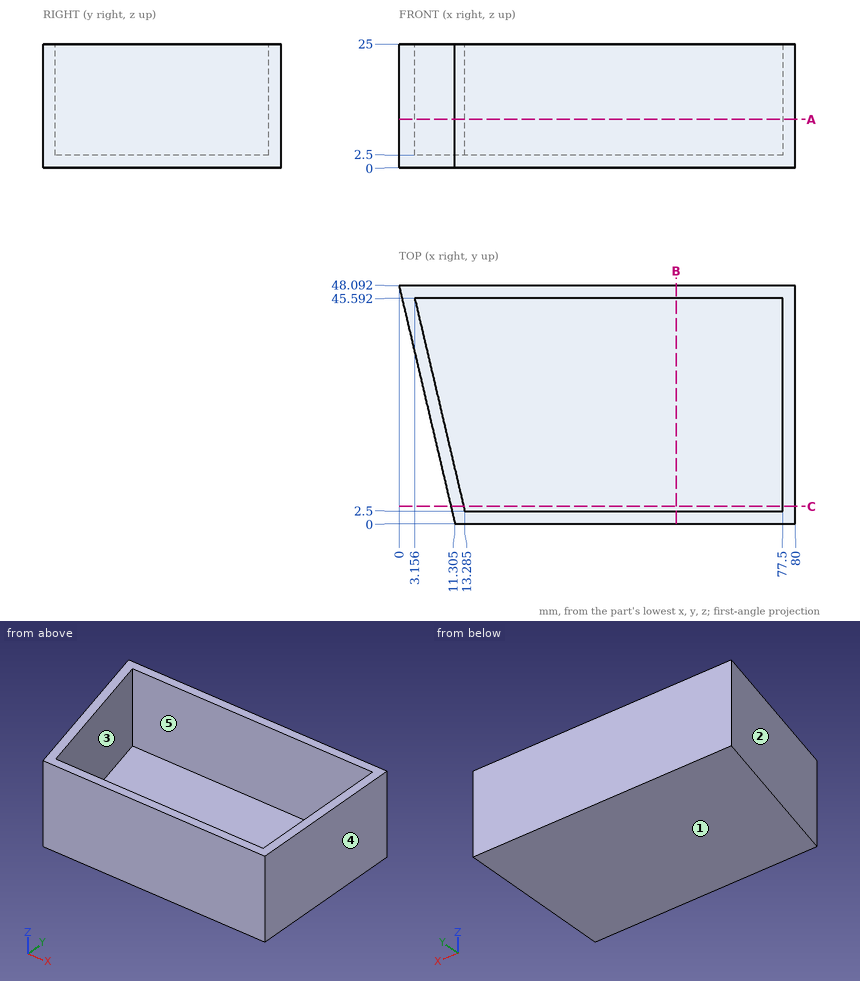
Print and shaded views of the part. All mm, measured from the part's lowest x, y and z. A direction names the side the tool comes from. Coordinates: 2 decimals unless noted, no trailing zeros. Write each loop counter-clockwise with the first axis right and the second up, starting at its lowest first coordinate (ties: lowest second). Pieces come first, ordered by that corner, then holes. Notation, with made-up numbers: M 17,81.25 L 65,81.25 A32 ccw 65,118.25 Z; hole C 12.25,48.5 d7. An arc over 180 degrees is marked long. Return JSON: item names as keys, results as strings.
1. Saw through at C-C, the plane y = 3.5. Write the cut outline in (x, z).
Determined:
{"outline": "M 10.48,0 L 80,0 L 80,25 L 77.5,25 L 77.5,2.5 L 13.05,2.5 L 13.05,25 L 10.48,25 Z"}
2. Flat gauge pins, fed straight in: pin 1 Ø10 at (y, z) = (36, 8) entering from -X; pin 2 Ø13 at (x, y) = (47, 33) entering from +Z. Where does each tip first touch, or does it go through?
Determined:
{"pin 1": "x = 1.67", "pin 2": "z = 2.5"}
3. Saw through at A-A, the plane z = 9.75. Write the cut outline in (x, y) (1 decimal).
Determined:
{"outline": "M 0,48.1 L 11.3,0 L 80,0 L 80,48.1 Z; hole M 3.2,45.6 L 13.3,2.5 L 77.5,2.5 L 77.5,45.6 Z"}
4. Saw through at B-B, the plane x = 56. Write the cut outline in (y, z), then the cut area to 3 significant figures.
Determined:
{"outline": "M 0,0 L 48.09,0 L 48.09,25 L 45.59,25 L 45.59,2.5 L 2.5,2.5 L 2.5,25 L 0,25 Z", "area": "233 mm²"}
5. Pull direction Y, two halves, no side cores. Call the marked faces 1, 2 and 3: pulls with the +Y half, pulls with the -Y half, needs draft (parallel to the pull), parting line crosses it, or undercut.
Determined:
{"face 1": "needs draft", "face 2": "pulls with the -Y half", "face 3": "undercut"}
6. Probe L1, parallel to Y at x = 74, z = 13; L2, parallel to Z at x = 12.5, y = 40; L3, parallel to X at y = 38, z = 9.75. List the from-to ranges inside material, lowest first.
Determined:
{"L1": "0 to 2.5, 45.59 to 48.09", "L2": "0 to 2.5", "L3": "2.37 to 4.94, 77.5 to 80"}
7. 3-axis set-ups, long thin cutter, end or side, ignore diameter. For the marked faces 4 and 5: which of +Z, -Z, +X, -X, +Y, -Y reach the whole face in a straight line?
Determined:
{"face 4": "+Z, -Z, +X, +Y, -Y", "face 5": "+Z"}
